```python
from build123d import *

# Parameters (mm, degrees)
F0_R     = 9.6
F1_DEPTH = 6


# Not quite as in the source:
# - ends of sketch curves that miss each other by under 0.0002 mm in the source are joined


with BuildPart() as f1:
    # F0 (on Front) → F1 (new body)
    with BuildSketch(Plane.XZ):
        with BuildLine():
            Line((-98.148557, 288.055726), (-98.148557, -287.944274))
            Line((-98.148557, -287.944274), (61.451443, -287.944274))
            ThreePointArc((61.451443, -287.944274), (90.8786929022, -275.1012880869), (96.4420569386, -243.4792343499))
            ThreePointArc((96.4420569386, -243.4792343499), (1.8673791595, 8.8528531517), (-32.087896312, 276.178294007))
            ThreePointArc((-32.087896312, 276.178294007), (-35.6454351808, 284.5842316136), (-44.087271, 288.055726))
            Line((-44.087271, 288.055726), (-98.148557, 288.055726))
        make_face()
        with BuildLine():
            ThreePointArc((-59.9885571325, -200.2110509435), (-29.1876571231, -155.9830655412), (16.7239738658, -127.7530766274))
            ThreePointArc((16.7239738658, -127.7530766274), (25.780399848, -128.1300293864), (31.9895542757, -134.7336148939))
            ThreePointArc((31.9895542757, -134.7336148939), (43.0295184538, -162.3758186302), (54.7647919037, -189.7300795987))
            ThreePointArc((54.7647919037, -189.7300795987), (54.7194507021, -199.5712496832), (47.3282871338, -206.0690474345))
            ThreePointArc((47.3282871338, -206.0690474345), (20.885121351, -226.2854831503), (13.9494494618, -258.8406940781))
            ThreePointArc((13.9494494618, -258.8406940781), (11.1483451659, -268.4168923847), (2.073951, -272.564799))
            Line((2.073951, -272.564799), (-48.948557, -272.564799))
            ThreePointArc((-48.948557, -272.564799), (-57.4338383742, -269.0500803742), (-60.948557, -260.564799))
            Line((-60.948557, -260.564799), (-60.948557, -204.914071))
            ThreePointArc((-60.948557, -204.914071), (-60.7061077935, -202.514071138), (-59.9885571325, -200.2110509435))
        make_face(mode=Mode.SUBTRACT)
        with BuildLine():
            ThreePointArc((-31.3094104055, 99.2474937685), (-30.7081992917, 96.8404508863), (-30.506005, 94.367714))
            ThreePointArc((-30.506005, 94.367714), (-11.0707369719, 1.2206915156), (15.8236014105, -90.0524808608))
            ThreePointArc((15.8236014105, -90.0524808608), (15.2706893662, -99.1138555668), (8.5302342503, -105.1950136941))
            ThreePointArc((8.5302342503, -105.1950136941), (-17.6222584193, -117.4699279564), (-41.0628425771, -134.3567693381))
            ThreePointArc((-41.0628425771, -134.3567693381), (-53.9170288848, -136.2346849428), (-60.948557, -125.311577))
            Line((-60.948557, -125.311577), (-60.948557, 94.367714))
            ThreePointArc((-60.948557, 94.367714), (-48.2000178863, 109.3867957083), (-31.3094104055, 99.2474937685))
        make_face(mode=Mode.SUBTRACT)
        with Locations((61.451443, -251.944274)):
            Circle(F0_R, mode=Mode.SUBTRACT)
    extrude(amount=F1_DEPTH)


solid = f1.part
```
CAD build for the part. Positions are in the model's coordinates, mm. A direction names the side the tool comes from. Round coordinates to 2 decimals unless told otherwise and drop trailing zeros. Order: outer loops, then holes, each group sorted by start corner. A loop starts at its lowest first (then second) coordinate and runs counter-clockwise, first axis right, second up. Notation, with made-up numbers: (73, -40) - (130, -40) arc R17 ccw to (130, -27) - close; hole circle Ø6 at (73, 26.5). An arc over 180 degrees is marked (long way). Use CSV: the item, a comma, the result in double quotes. Start each with the question number.
1) Two-plate mould, pull along Z, no slides. Class faces 3 (the cylindrical face through (-29.74, -2.96, -156.51)), 4 (the flat face through (-67, 0, 4)), 5 (the cylindrical face through (-35.55, -2.96, 284.49)): pulls with the +Z half, pulls with the -Z half, needs draft (parallel to the pull), parting line crosses it, or undercut.
2) Pin check, flat tips, straight feed: pin 1 Ø1.5 at (y, z) = (-3.5, -191.5) entering from +X; pin 2 Ø3 at (x, y) = (-8, -4.5) entering from -Z. Stop position of each tip, or through.
3) Saw through at A-A (x = 38). List the corners of the cut face in (y, z), and give its area (3 significant figures).
4) Wall check: L1, parallel to Z at x = -51.5, y = -5.1; L2, parallel to Z at x = -52.5, y = -5.35; L3, parallel to X at y = -1.6, z = -153. Give the ranges that are in metal, low to high. Write a range as [from, to].
5) Saw through at C-C (z = -80). List the corners of the cut face in (x, y), and give its area (3 significant figures).
6) Saw through at D-D (z = 235). List the corners of the cut face in (x, y).
7) Tool access for faces 1 (the cylindrical face through (-11.395, -2.958, 2.513)), 2 (the cylindrical face through (2.781, -2.958, 5.184)): list every direction of +Z, -Z, +X, -X, +Y, -Y with a clear straight run to the whole face (end or side of a thin tool).
8) Saw through at B-B (y = -2.8). List the corners of the cut face in (x, z).
Values follow:
1,face 3,"undercut"
1,face 4,"needs draft"
1,face 5,"pulls with the +Z half"
2,pin 1,"stops at x = 71.68"
2,pin 2,"stops at z = -287.94"
3,outline,"(-6, -287.94) - (0, -287.94) - (0, -210.06) - (-6, -210.06) - close; (-6, -150.03) - (0, -150.03) - (0, -109.72) - (-6, -109.72) - close"
3,area,"709 mm2"
4,L1,"z = [-287.94, -272.29], [-183.64, -137.04], [108.45, 288.06]"
4,L2,"z = [-287.94, -272.03], [-185.32, -136.77], [108, 288.06]"
4,L3,"x = [-98.15, -25.92], [39.19, 54.74]"
5,outline,"(-98.15, -6) - (-60.95, -6) - (-60.95, 0) - (-98.15, 0) - close; (12.46, -6) - (27.63, -6) - (27.63, 0) - (12.46, 0) - close"
5,area,"314 mm2"
6,outline,"(-98.15, -6) - (-30.94, -6) - (-30.94, 0) - (-98.15, 0) - close"
7,face 1,"+Y, -Y"
7,face 2,"+Z, +X, +Y, -Y"
8,outline,"(-98.15, -287.94) - (61.45, -287.94) arc R33.95 ccw to (96.44, -243.48) arc R1162.86 cw to (-32.09, 276.18) arc R12 ccw to (-44.09, 288.06) - (-98.15, 288.06) - close; hole (-60.95, -260.56) arc R12 ccw to (-48.95, -272.56) - (2.07, -272.56) arc R12 ccw to (13.95, -258.84) arc R48 cw to (47.33, -206.07) arc R12 ccw to (54.76, -189.73) arc R1177.26 cw to (31.99, -134.73) arc R12 ccw to (16.72, -127.75) arc R132 ccw to (-59.99, -200.21) arc R12 ccw to (-60.95, -204.91) - close; hole (-60.95, -125.31) arc R12 ccw to (-41.06, -134.36) arc R156 cw to (8.53, -105.2) arc R12 ccw to (15.82, -90.05) arc R1177.26 cw to (-30.51, 94.37) arc R15.22 ccw to (-60.95, 94.37) - close; hole circle Ø19.2 at (61.45, -251.94)"
